Answer from the drawing. Dimensions are ordinates in mm from the lowest x, y and z of the part. A direction names the side the tool comes from. Give positions to 0.01 mm unless a question says otherwise; leave off trailing zeros. Loops run counter-clockwise (first coordinate to the right, second up) from the corner with the lowest first, then second, coordinate; pieces in that order, holes last. Notation, with made-up numbers: (54.25, 12) - (89.25, 12) arc R23 cw to (89.25, 41) - close; hole circle Ø3 at (11.25, 67). An arc over 180 degrees is marked (long way). Answer as CSV lines item,"result". Start each with the question number.
1) For a pull along X with two mould halves and no side action, classify the marked faces 4, 5 and 6 as pulls with the +X half, pulls with the -X half, needs draft (parallel to the pull), parting line crosses it, or undercut.
2) For the marked faces 1, 2 and 3, determine the directions among +Z, -Z, +X, -X, +Y, -Y from which every point of the face is accessible in a straight line to the end or side of a thin tool.
3) A cutting plane is placed at D-D (x = 169). Determine the outline of the cut face in (y, z).
4) A cutting plane is placed at A-A (y = 144). Determine the outline of the cut face in (x, z), and give its area (3 significant figures).
5) A cutting plane is placed at C-C (x = 138.5). Determine the outline of the cut face in (y, z), and give its area (3 significant figures).
6) A cutting plane is placed at B-B (z = 10). Determine the outline of the cut face in (x, y), and give its area (3 significant figures).
7) Find the intervals of material crossed by line 1 along X through (y, z) = (150, 3.75) (1 decimal); line 2 along X through (y, z) = (66, 0.5); line 3 along Y through (x, z) = (75, 10.75), in increasing order.
8) Flat-ended cylindrical pins translate along their axes: pin 1 (3 mm diameter, centred on y = 24.5, z = 4, fed in from -X); pin 2 (3 mm diameter, centred on x = 119, y = 104, fed in from -Z); pin 3 (3 mm diameter, centred on x = 49, z = 10, fed in from +Y); pin 4 (1.5 mm diameter, centred on x = 178, z = 9.5, fed in from -Y). Find the tip coordinate at first contact, or state that the pin passes through.
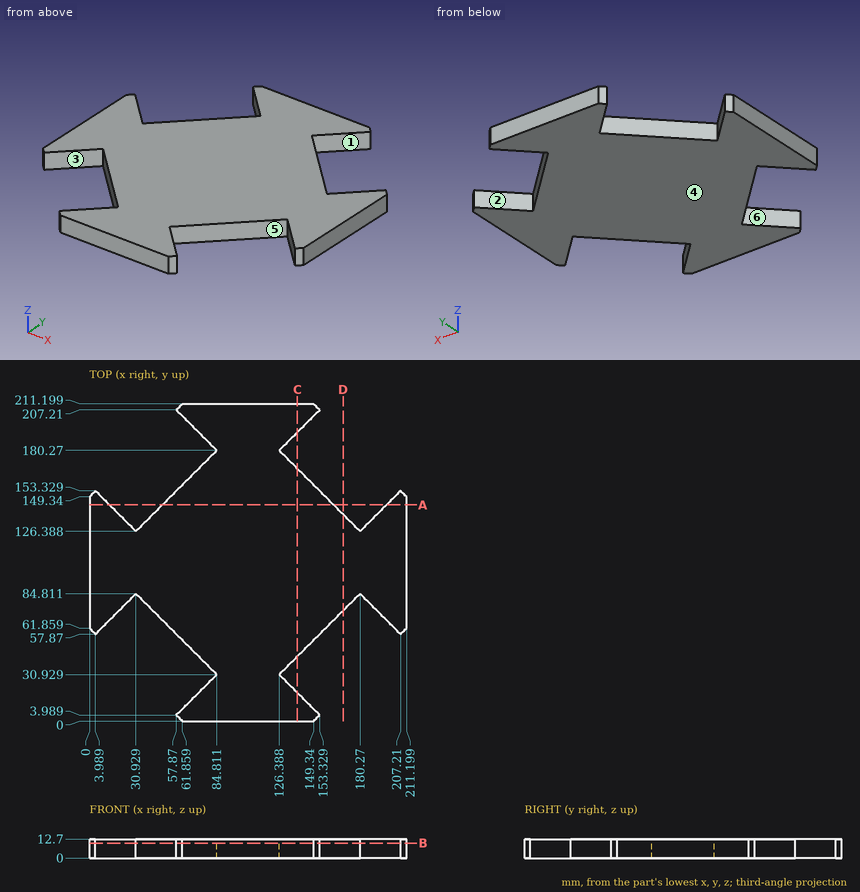
Ans:
1,face 4,"needs draft"
1,face 5,"undercut"
1,face 6,"pulls with the -X half"
2,face 1,"+Z, -Z, +X"
2,face 2,"+Z, -Z, +Y"
2,face 3,"+Z, -Z, -Y"
3,outline,"(73.54, 0) - (137.66, 0) - (137.66, 12.7) - (73.54, 12.7) - close"
4,outline,"(0, 0) - (13.32, 0) - (13.32, 12.7) - (0, 12.7) - close; (48.54, 0) - (162.66, 0) - (162.66, 12.7) - (48.54, 12.7) - close; (197.88, 0) - (211.2, 0) - (211.2, 12.7) - (197.88, 12.7) - close"
4,area,"1,790 mm2"
5,outline,"(0, 0) - (18.82, 0) - (18.82, 12.7) - (0, 12.7) - close; (43.04, 0) - (168.16, 0) - (168.16, 12.7) - (43.04, 12.7) - close; (192.38, 0) - (211.2, 0) - (211.2, 12.7) - (192.38, 12.7) - close"
5,area,"2,070 mm2"
6,outline,"(0, 61.86) - (3.99, 57.87) - (30.93, 84.81) - (84.81, 30.93) - (57.87, 3.99) - (61.86, 0) - (149.34, 0) - (153.33, 3.99) - (126.39, 30.93) - (180.27, 84.81) - (207.21, 57.87) - (211.2, 61.86) - (211.2, 149.34) - (207.21, 153.33) - (180.27, 126.39) - (126.39, 180.27) - (153.33, 207.21) - (149.34, 211.2) - (61.86, 211.2) - (57.87, 207.21) - (84.81, 180.27) - (30.93, 126.39) - (3.99, 153.33) - (0, 149.34) - close"
6,area,"25,300 mm2"
7,line 1,"0.7 to 7.3, 54.5 to 156.7, 203.9 to 210.5"
7,line 2,"0 to 12.12, 49.74 to 161.46, 199.08 to 211.2"
7,line 3,"0 to 21.12, 40.74 to 170.46, 190.08 to 211.2"
8,pin 1,"x = 76.88"
8,pin 2,"z = 0"
8,pin 3,"y = 145.96"
8,pin 4,"y = 81.79"
